Could you check a few things on this model? Use its own coordinates, in mm. Face numbers are marked on the shaded views. A direction names the side the tool comes from. Round coordinates to 2 decimals unless told otherwise and drop trailing zeros. Loops run counter-clockwise (first coordinate to the right, second up) from the corner with the lowest first, then second, coordinate; pieces in that order, holes last. Notation, with made-up numbers: M 50.25,5 L 107.25,5 A20 cw 107.25,40 Z; hole C 54,0.25 d2. An arc over 180 degrees is marked long. Return JSON: item names as keys, results as strings. Group by question number.
```python
from build123d import *

# Parameters (mm, degrees)
BOSS_EXTRUDE3_DEPTH = 320
SKETCH8_W           = 15
SKETCH8_H           = 111
CUT_EXTRUDE4_DEPTH  = 321.702354216
BOSS_EXTRUDE5_DEPTH = 140
SKETCH4_W           = 58
SKETCH4_H           = 63
SKETCH4_R           = 3.8
BOSS_EXTRUDE4_DEPTH = 6
BOSS_EXTRUDE6_DEPTH = 15
CUT_EXTRUDE5_DEPTH  = 226.279401317
SKETCH12_R          = 6.8
CUT_EXTRUDE6_DEPTH  = 3


with BuildPart() as part:
    # Sketch1 → Boss-Extrude3 (new body)
    with BuildSketch(Plane(origin=(0, 0, 0), x_dir=(1, 0, 0), z_dir=(0, 1, 0))):
        Polygon((0, 0), (0, 15), (15, 0), align=None)
    extrude(amount=BOSS_EXTRUDE3_DEPTH)

    # Sketch8 → Cut-Extrude4 (cut, through all)
    with BuildSketch(Plane.XY):
        with Locations((7.5, 264.5)):
            Rectangle(SKETCH8_W, SKETCH8_H)
    extrude(amount=-CUT_EXTRUDE4_DEPTH, mode=Mode.SUBTRACT)

    # Sketch9 → Boss-Extrude5 (add)
    with BuildSketch(Plane.XZ):
        Polygon((-3, -22.242640687), (-3, 3), (22.242640687, 3), align=None)
    extrude(amount=-BOSS_EXTRUDE5_DEPTH)

    # Sketch4 → Boss-Extrude4 (add)
    with BuildSketch(Plane.XZ):
        with Locations((26, -28.5)):
            Rectangle(SKETCH4_W, SKETCH4_H)
        with Locations(Location((45.59, -40.3, 0), (0, 0, 270))):
            Circle(SKETCH4_R, mode=Mode.SUBTRACT)
    extrude(amount=-BOSS_EXTRUDE4_DEPTH)

    # Sketch10 → Boss-Extrude6 (add)
    with BuildSketch(Plane(origin=(0, 6, 0), x_dir=(1, 0, 0), z_dir=(0, 1, 0))):
        Polygon((-3, 22.242640687), (7.606601718, 32.849242405), (32.849242405, 7.606601718), (22.242640687, -3), align=None)
    extrude(amount=BOSS_EXTRUDE6_DEPTH)

    # Sketch11 → Cut-Extrude5 (cut, through all)
    with BuildSketch(Plane(origin=(12.621320344, 0, 12.621320344), x_dir=(0.7071067811865477, 0, -0.7071067811865475), z_dir=(0.7071067811865475, 0, 0.7071067811865477))):
        with BuildLine():
            Line((13.606601718, 21), (28.606601718, 21))
            Line((28.606601718, 21), (28.606601718, 6))
            ThreePointArc((28.606601718, 6), (18, 10.393398282), (13.606601718, 21))
        make_face()
    extrude(amount=-CUT_EXTRUDE5_DEPTH, mode=Mode.SUBTRACT)

    # Sketch12 → Cut-Extrude6 (cut)
    with BuildSketch(Plane(origin=(0, 6, 0), x_dir=(1, 0, 0), z_dir=(0, 1, 0))):
        with Locations(Location((45.59, 40.3, 0), (0, 0, 270))):
            Circle(SKETCH12_R)
    extrude(amount=-CUT_EXTRUDE6_DEPTH, mode=Mode.SUBTRACT)


solid = part.part
```
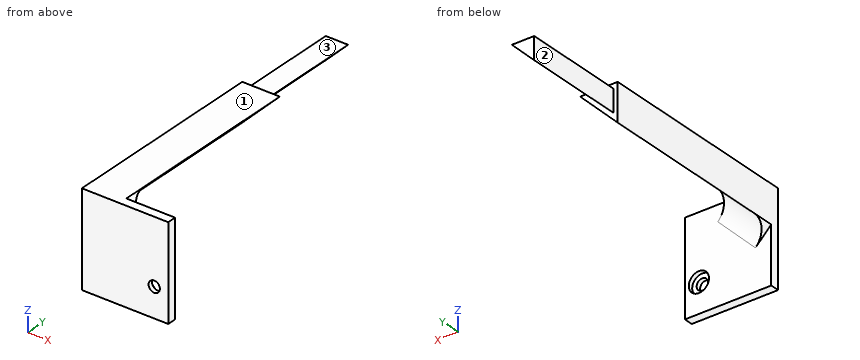
1. If we section it at A-A, the plane z = -40.3: Please give me the cut outline in (x, y).
2. If we section it at B-B, the plane x = 45.59: Please give me the cut outline in (y, z).
3. If we section it at C-C, the plane z = -50.5: Please give me the cut outline in (x, y), then the cut area to 3 significant figures.
4. I need wall thicknesses on probe 1 along X at (y, z) = (1.9, -40.3); probe 2 along X at (y, z) = (4.9, -40.3); probe 3 along Y at (x, z) = (4, -29.5). Which ranges of each line are inside material? Lowest first, please.
5. I'm going to push flat-ended pins straight in: pin 1 Ø4 at (x, y) = (6, 177.5) entering from -Z; pin 2 Ø3 at (x, z) = (35, -34) entering from +Y; pin 3 Ø7.5 at (y, z) = (175, -5) entering from -X. Where does each tip first touch, or does it pass through?
6. On a 3-axis mill with a long thin cutter (end or side, diameter ignored), from which of +Z, -Z, +X, -X, +Y, -Y can I reach the whole of each face in a straight line? I mean the marked faces 1, 2 and 3. Say none if no direction works.
7. If we section it at D-D, the plane y = 137: Please give me the cut outline in (x, z), then the cut area to 3 significant figures.
Geometry results:
{
 "1": {"outline": "M -3,0 L 41.79,0 L 41.79,3 L 38.79,3 L 38.79,6 L -3,6 Z; M 49.39,0 L 55,0 L 55,6 L 52.39,6 L 52.39,3 L 49.39,3 Z"},
 "2": {"outline": "M 0,-60 L 6,-60 L 6,-47.1 L 3,-47.1 L 3,-44.1 L 0,-44.1 Z; M 0,-36.5 L 3,-36.5 L 3,-33.5 L 6,-33.5 L 6,3 L 0,3 Z"},
 "3": {"outline": "M -3,0 L 55,0 L 55,6 L -3,6 Z", "area": "348 mm^2"},
 "4": {"probe 1": "-3 to 41.79, 49.39 to 55", "probe 2": "-3 to 38.79, 52.39 to 55", "probe 3": "0 to 6"},
 "5": {"pin 1": "z = -11", "pin 2": "y = 6", "pin 3": "x = 0"},
 "6": {"face 1": "+Z, +X, -X, +Y, -Y", "face 2": "+Z, -Z, -X, +Y", "face 3": "+Z, +X, -X, +Y"},
 "7": {"outline": "M -3,-22.24 L 22.24,3 L -3,3 Z", "area": "319 mm^2"}
}
